Work out the finished part from the listing and answer in its coordinate system (mm). Face numbers are marked on the shaded views. A direction names the side the tool comes from. Coordinates: 2 decimals unless noted, no trailing zeros. Loops run counter-clockwise (first coordinate to the right, second up) from the corner with the lowest first, then second, coordinate; pieces in that order, holes last. Notation, with made-up numbers: (76.25, -25.75) -> (134.25, -25.75) arc R27 cw to (134.25, 2.25) -> close; hole circle Ø9 at (40.5, -21). An arc over 180 degrees is marked (long way). Answer as CSV lines item,"result".
```python
from build123d import *

# Parameters (mm, degrees)
SKETCH2_R          = 3.175
CUT_EXTRUDE1_DEPTH = 101.6
SKETCH3_W          = 2.54
SKETCH3_H          = 14.827996595
SKETCH3_H_2        = 14.256172231
CUT_EXTRUDE2_DEPTH = 12.7
SKETCH4_R          = 3.2639
CUT_EXTRUDE3_DEPTH = 124.410028215


with BuildPart() as part:
    # Sketch1 → Revolve2 (revolve)
    with BuildSketch(Plane.XY, mode=Mode.PRIVATE) as revolve2_sk:
        Polygon((-12.7, 20.32), (-12.7, 12.7), (119.38, 12.7), (119.38, 20.32), (114.3, 20.32), (114.3, 25.4), (0, 25.4), (0, 20.32), align=None)
    revolve(revolve2_sk.sketch.rotate(Axis((-12.7, 12.7, 0), (1, 0, 0)), 90), axis=Axis((-12.7, 12.7, 0), (1, 0, 0)))

    # Sketch2 → Cut-Extrude1 (cut)
    with BuildSketch(Plane(origin=(119.38, 0, 0), x_dir=(0, 0, -1), z_dir=(1, 0, 0))):
        with Locations((0, 12.7)):
            Circle(SKETCH2_R)
    extrude(amount=-CUT_EXTRUDE1_DEPTH, mode=Mode.SUBTRACT)

    # Sketch3 → Cut-Extrude2 (cut)
    with BuildSketch(Plane.ZY.offset(12.7)):
        with Locations((-6.82625, 12.906001702)):
            Rectangle(SKETCH3_W, SKETCH3_H)
        with Locations((6.82625, 13.191913884)):
            Rectangle(SKETCH3_W, SKETCH3_H_2)
    extrude(amount=-CUT_EXTRUDE2_DEPTH, mode=Mode.SUBTRACT)

    # Sketch4 → Cut-Extrude3 (cut, through all)
    with BuildSketch(Plane.XY.offset(5.55625)):
        with Locations((-6.35, 12.834641497)):
            Circle(SKETCH4_R)
    extrude(amount=-CUT_EXTRUDE3_DEPTH, mode=Mode.SUBTRACT)


solid = part.part
```
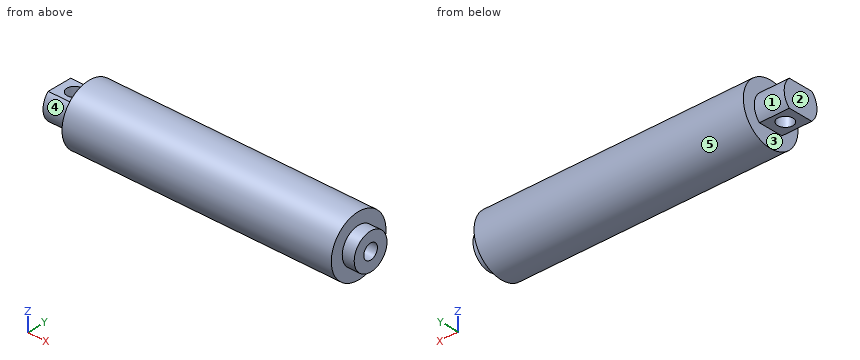
(1) A cutting plane is placed at B-B, the plane z = 0. Write down the section's boundary in (x, y) (3 decimals).
Computed values:
outline,"(-12.7, 5.08) -> (0, 5.08) -> (0, 0) -> (114.3, 0) -> (114.3, 5.08) -> (119.38, 5.08) -> (119.38, 9.525) -> (17.78, 9.525) -> (17.78, 15.875) -> (119.38, 15.875) -> (119.38, 20.32) -> (114.3, 20.32) -> (114.3, 25.4) -> (0, 25.4) -> (0, 20.32) -> (-12.7, 20.32) -> close; hole circle Ø6.528 at (-6.35, 12.835)"
(2) A cutting plane is placed at A-A, the plane x = -6.35. Write down the section's boundary in (y, z).
Computed values:
outline,"(7.49, -5.56) -> (9.57, -5.56) -> (9.57, 5.56) -> (7.49, 5.56) arc R7.62 ccw to start; (16.1, -5.56) -> (17.91, -5.56) arc R7.62 ccw to (17.91, 5.56) -> (16.1, 5.56) -> close"
(3) Consider line 1 along Y through (x, z) = (51, 0) (3 decimals); line 2 along Y through (x, z) = (-6.35, -0.5); line 3 along X through (y, z) = (12.5, 2.25). Determine where each line is inside the solid, lowest interval first.
Computed values:
line 1,"0 to 9.525, 15.875 to 25.4"
line 2,"5.1 to 9.57, 16.1 to 20.3"
line 3,"-12.7 to -9.6, -3.1 to 17.78"
(4) Flat-ended cylindrical pins translate along their axes: pin 1 Ø1.5 at (x, z) = (87, -4.5) entering from +Y; pin 2 Ø4 at (y, z) = (12.7, 0) entering from +X; pin 3 Ø8.5 at (x, y) = (-4, 10.5) entering from +Z. Find the tip coordinate at first contact, or state that the pin passes through.
Computed values:
pin 1,"y = 24.83"
pin 2,"x = 17.78"
pin 3,"z = 12.68"
(5) A cutting plane is placed at D-D, the plane x = 87. Write down the section's boundary in (y, z) (3 decimals), and give its area (3 significant figures).
Computed values:
outline,"circle Ø25.4 at (12.7, 0); hole circle Ø6.35 at (12.7, 0)"
area,"475 mm2"
(6) Which of the six approach directions +Z, -Z, +X, -X, +Y, -Y give full straight-line access (tool end or side, diameter ignored) to the marked faces 1, 2, 3, 4 and 5?
Computed values:
face 1,"-X, +Y"
face 2,"+Z, -Z, -X, +Y, -Y"
face 3,"-X"
face 4,"-X, -Y"
face 5,"+X, -X"
(7) A cutting plane is placed at C-C, the plane y = 14.25. Write down the section's boundary in (x, z), and give its area (3 significant figures).
Computed values:
outline,"(-12.7, -5.56) -> (-9.29, -5.56) -> (-9.29, 5.56) -> (-12.7, 5.56) -> close; (-3.41, -5.56) -> (0, -5.56) -> (0, -12.61) -> (114.3, -12.61) -> (114.3, -7.46) -> (119.38, -7.46) -> (119.38, -2.77) -> (17.78, -2.77) -> (17.78, 2.77) -> (119.38, 2.77) -> (119.38, 7.46) -> (114.3, 7.46) -> (114.3, 12.61) -> (0, 12.61) -> (0, 5.56) -> (-3.41, 5.56) -> close"
area,"2,470 mm2"
